from build123d import *

# Parameters (mm, degrees)
SKETCH_1_R      = 1.6
EXTRUDE_1_DEPTH = 3


with BuildPart() as part:
    # 草图1 → 凸台-拉伸1 (new body)
    with BuildSketch(Plane.XY):
        Polygon((0, 0), (55, 0), (55, -15), (15, -55), (0, -55), align=None)
        with Locations((3.75, -50)):
            Circle(SKETCH_1_R, mode=Mode.SUBTRACT)
        with Locations(Location((11.25, -50, 0), (0, 0, 180))):
            Circle(SKETCH_1_R, mode=Mode.SUBTRACT)
        with Locations((11.25, -40)):
            Circle(SKETCH_1_R, mode=Mode.SUBTRACT)
        with Locations(Location((3.75, -40, 0), (0, 0, 180))):
            Circle(SKETCH_1_R, mode=Mode.SUBTRACT)
        with Locations((50, -3.75)):
            Circle(SKETCH_1_R, mode=Mode.SUBTRACT)
        with Locations(Location((50, -11.25, 0), (0, 0, 180))):
            Circle(SKETCH_1_R, mode=Mode.SUBTRACT)
        with Locations((40, -11.25)):
            Circle(SKETCH_1_R, mode=Mode.SUBTRACT)
        with Locations(Location((40, -3.75, 0), (0, 0, 180))):
            Circle(SKETCH_1_R, mode=Mode.SUBTRACT)
        Polygon((16.5, -16.5), (16.5, -40.772077939), (40.772077939, -16.5), align=None, mode=Mode.SUBTRACT)
        Polygon((3.5, -3.5), (11.5, -3.5), (3.5, -11.5), align=None, mode=Mode.SUBTRACT)
        Polygon((15.5, -3.5), (7.5, -11.5), (15.5, -11.5), align=None, mode=Mode.SUBTRACT)
    extrude(amount=EXTRUDE_1_DEPTH)


solid = part.part
Geometry: final body of the model. Coordinates: model frame, mm. A direction names the side the tool comes from. Round coordinates to 2 decimals unless told otherwise and drop trailing zeros. Loops run counter-clockwise (first coordinate to the right, second up) from the corner with the lowest first, then second, coordinate; pieces in that order, holes last.
Q1. Section B-B on z = 2.35. State how many separate pieces and enclosed holes the cut face has, plus the area to 3 significant figures.
Q2. Section D-D on x = 21.5. Return loops of the section in (y, z), plus the area to 3 significant figures.
Q3. Section C-C on y = -40. Return loops of the section in (x, z).
Q4. Pin query (flat end, axial travel): P1, Ø1, axis at y = -16, z = 0.5, coming from the +X side; P2, Ø1.5, axis at x = 32.5, z = 2, coming from the -Y side; P3, Ø6, axis at x = 9.5, y = -36, coming from the -Z side; P4, Ø3, axis at x = 50, y = -3.75, coming from the -Z side. Return the tip coordinate at first contact, or that it passes through.
Q5. Pull-direction query (Y, two-part tool) for faces 3 (the cylindrical face through (48.474, -11.731, 1.479)), 4 (the flat face through (35, -35, 1)), 5 (the flat face through (22, -15, 0)); classes: released by +Y, released by -Y, zero draft, split by the parting line, or undercut.
Q6. Access query for faces 1 (the flat face through (0, -28, 1)), 2 (the flat face through (8, -7, 1)). Directions: +Z, -Z, +X, -X, +Y, -Y. A direction counts if a zero-diameter tool reaches every point of the face in a straight line with its end or side. Return the directions, or none.
Q7. Section A-A on x = 50. Return loops of the section in (y, z).
Q8. Material intervals for L1, parallel to X at y = -39.5, z = 2.85; L2, parallel to X at y = -12, z = 1.6; L3, parallel to X at y = -11, z = 0.5, sorted ascending.
Evaluation:
1. separate pieces: 1
1. enclosed holes: 11
1. area: 1,800 mm2
2. outline: (-48.5, 0) - (-35.77, 0) - (-35.77, 3) - (-48.5, 3) - close; (-16.5, 0) - (0, 0) - (0, 3) - (-16.5, 3) - close
2. area: 87.7 mm2
3. outline: (0, 0) - (2.15, 0) - (2.15, 3) - (0, 3) - close; (5.35, 0) - (9.65, 0) - (9.65, 3) - (5.35, 3) - close; (12.85, 0) - (16.5, 0) - (16.5, 3) - (12.85, 3) - close; (17.27, 0) - (30, 0) - (30, 3) - (17.27, 3) - close
4. P1: stops at x = 54.5
4. P2: stops at y = -38.25
4. P3: stops at z = 0
4. P4: passes through
5. face 3: undercut
5. face 4: released by -Y
5. face 5: zero draft
6. face 1: +Z, -Z, -X, +Y, -Y
6. face 2: +Z, -Z
7. outline: (-20, 0) - (-12.85, 0) - (-12.85, 3) - (-20, 3) - close; (-9.65, 0) - (-5.35, 0) - (-5.35, 3) - (-9.65, 3) - close; (-2.15, 0) - (0, 0) - (0, 3) - (-2.15, 3) - close
8. L1: x = 0 to 2.23, 5.27 to 9.73, 12.77 to 16.5, 17.77 to 30.5
8. L2: x = 0 to 38.59, 41.41 to 48.59, 51.41 to 55
8. L3: x = 0 to 3.5, 4 to 8, 15.5 to 38.42, 41.58 to 48.42, 51.58 to 55
